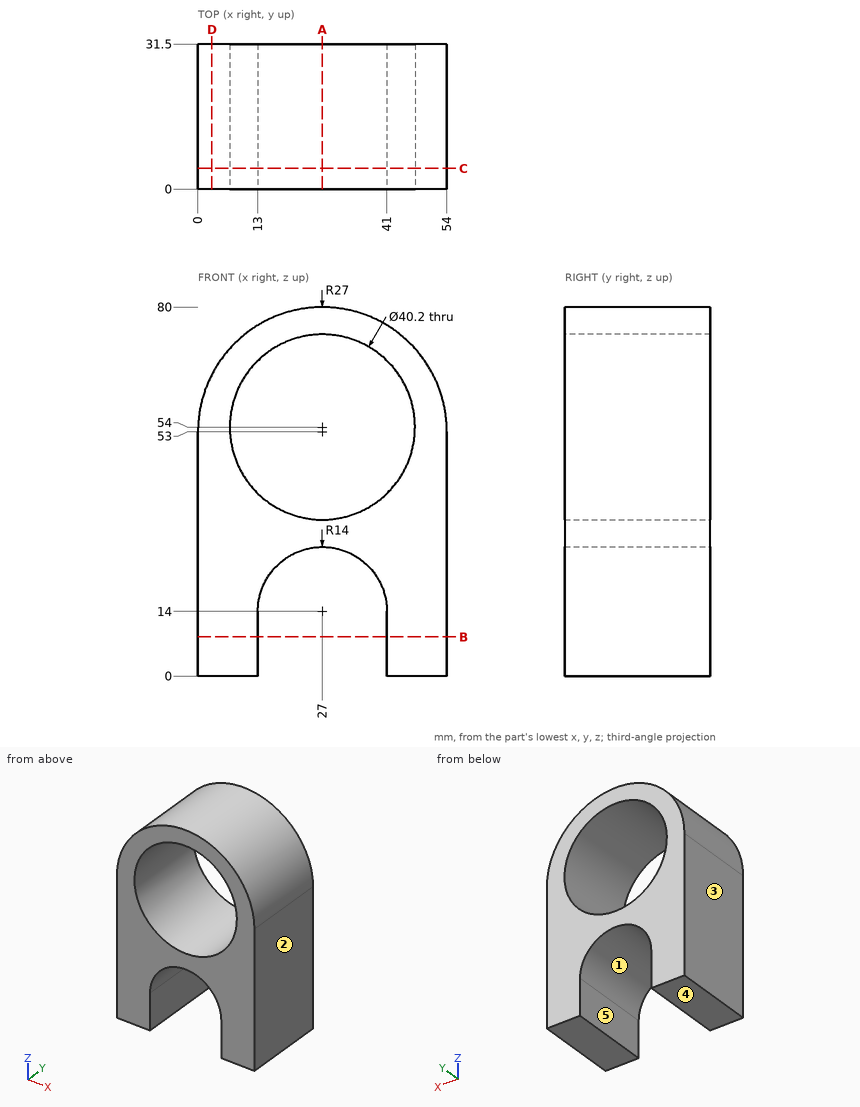
Can you work these out from the drawing? Everything is in mm from the part's minimum corner. A direction names the side the tool comes from. Coordinates: 2 decimals unless noted, no trailing zeros. Loops run counter-clockwise (first coordinate to the right, second up) from the corner with the lowest first, then second, coordinate; pieces in that order, holes last.
1) Imagine slicing it at A-A (x = 27). List the corners of the cut face in (y, z) for me.
Reported:
outline: (0, 28) - (31.5, 28) - (31.5, 33.9) - (0, 33.9) - close; (0, 74.1) - (31.5, 74.1) - (31.5, 80) - (0, 80) - close
2) Please list where these lines run through material, in increasing order: line 1 along X through (y, z) = (7.5, 54); line 2 along X through (y, z) = (6.5, 50); line 3 along Z through (x, y) = (9, 11.5).
Reported:
line 1: x = 0.02 to 6.9, 47.1 to 53.98
line 2: x = 0 to 7.3, 46.7 to 54
line 3: z = 0 to 45.06, 62.94 to 73.12
3) Thinking about a two-plate mould opening in X: for the marked faces 1, 2 and 3, which applies, released by +X, released by -X, zero draft, split by the parting line, or undercut?
Reported:
face 1: undercut
face 2: released by +X
face 3: released by -X
4) Will these pins go through, and if not, where does the flat tip stop? pin 1 Ø1.5 at (y, z) = (21.5, 67.5) entering from -X; pin 2 Ø12 at (x, z) = (27.5, 19.5) entering from +Y; pin 3 Ø8 at (x, y) = (30, 20) entering from +Z; pin 4 Ø3 at (x, y) = (36.5, 13) entering from -Z.
Reported:
pin 1: stops at x = 3.76
pin 2: passes through
pin 3: stops at z = 80
pin 4: stops at z = 22.66
5) Which directions (+Z, -Z, +X, -X, +Y, -Y) give clear straight access to the entire face, cutting with the end or side of a thin tool? Please do the marked faces 4 and 5.
Reported:
face 4: -Z, +X, -X, +Y, -Y
face 5: -Z, +Y, -Y
6) Imagine slicing it at C-C (y = 4.5). List the corners of the cut face in (x, z) for me.
Reported:
outline: (0, 0) - (13, 0) - (13, 14) arc R14 cw to (41, 14) - (41, 0) - (54, 0) - (54, 53) arc R27 ccw to (0, 53) - close; hole circle Ø40.2 at (27, 54)
7) Imagine slicing it at B-B (z = 8.5). List the corners of the cut face in (x, y) for me.
Reported:
outline: (0, 0) - (13, 0) - (13, 31.5) - (0, 31.5) - close; (41, 0) - (54, 0) - (54, 31.5) - (41, 31.5) - close
8) Imagine slicing it at D-D (x = 3). List the corners of the cut face in (y, z) for me, and give its area (3 significant figures).
Reported:
outline: (0, 0) - (31.5, 0) - (31.5, 65.37) - (0, 65.37) - close
area: 2,060 mm2
